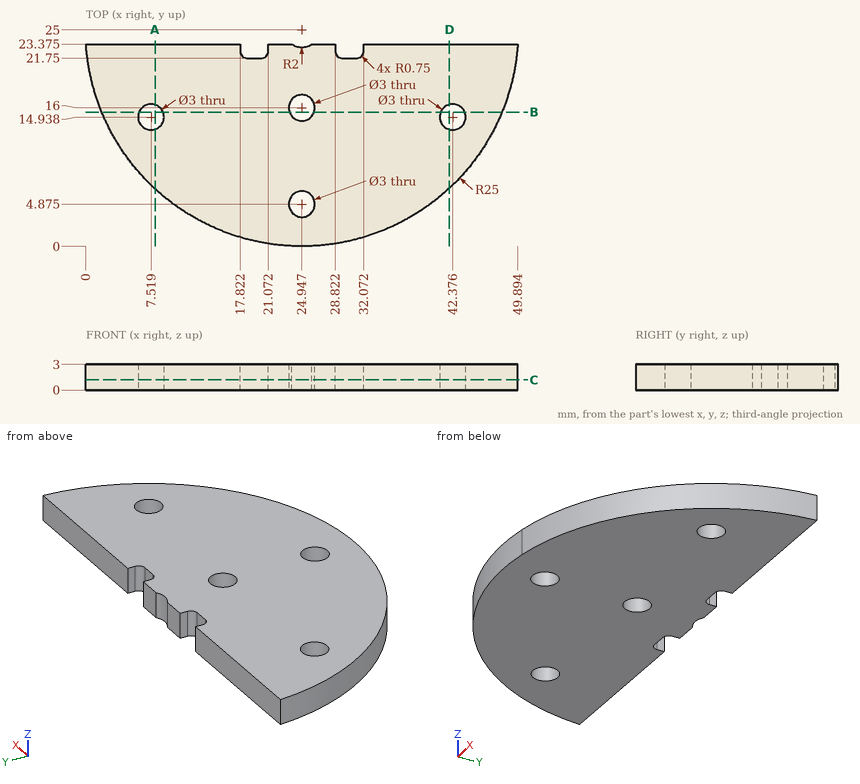
Here's the drawing with two shaded views (mm, measured from the low corner). I have some questions. Give positions to 0.01 mm unless a question says otherwise; leave off trailing zeros. Loops run counter-clockwise (first coordinate to the right, second up) from the corner with the lowest first, then second, coordinate; pieces in that order, holes last. Notation, with made-up numbers: (45.25, 13) -> (86.25, 13) arc R23 cw to (86.25, 28) -> close; hole circle Ø6 at (29, 77). An arc over 180 degrees is marked (long way). Answer as a JSON object with one key per item and string values. Group by question number.
Item 1: Imagine slicing it at B-B on y = 15.5. Write out the boundary of the cut face in (x, z) (1 decimal).
Item 2: Imagine slicing it at D-D on x = 42. Write out the boundary of the cut face in (y, z) (1 decimal).
Item 3: Imagine slicing it at A-A on x = 8. Write out the boundary of the cut face in (y, z) (1 decimal).
Item 4: I need wall thicknesses on L1, parallel to Y at x = 25, z = 2.7 (1 decimal); L2, parallel to X at y = 22, z = 2.6 (1 decimal); L3, parallel to Y at x = 42.5, z = 1.7 (1 decimal). Which ranges of each line are inside material? Lowest first, please.
Item 5: Imagine slicing it at C-C on z = 1.2. Give the number of separate pieces and of enclosed holes in the cut face.
Item 6: Will these pins go through, and if not, where does the flat tip stop? pin 1 (1 mm diameter, centred on x = 25, z = 2.5, fed in from +Y); pin 2 (0.7 mm diameter, centred on y = 23, z = 1, fed in from -X); pin 3 (3.5 mm diameter, centred on x = 24.95, y = 16, fed in from +Z); pin 4 (0.9 mm diameter, centred on x = 20, z = 1, fed in from +Y).
Answer list:
{
 "1": {"outline": "(1.8, 0) -> (6.1, 0) -> (6.1, 3) -> (1.8, 3) -> close; (8.9, 0) -> (23.5, 0) -> (23.5, 3) -> (8.9, 3) -> close; (26.4, 0) -> (41, 0) -> (41, 3) -> (26.4, 3) -> close; (43.8, 0) -> (48.1, 0) -> (48.1, 3) -> (43.8, 3) -> close"},
 "2": {"outline": "(6.7, 0) -> (13.5, 0) -> (13.5, 3) -> (6.7, 3) -> close; (16.4, 0) -> (23.4, 0) -> (23.4, 3) -> (16.4, 3) -> close"},
 "3": {"outline": "(6.6, 0) -> (13.5, 0) -> (13.5, 3) -> (6.6, 3) -> close; (16.4, 0) -> (23.4, 0) -> (23.4, 3) -> (16.4, 3) -> close"},
 "4": {"L1": "y = 0 to 3.4, 6.4 to 14.5, 17.5 to 23", "L2": "x = 0.1 to 18, 20.9 to 29, 31.9 to 49.8", "L3": "y = 7.2 to 13.4, 16.4 to 23.4"},
 "5": {"separate pieces": "1", "enclosed holes": "4"},
 "6": {"pin 1": "stops at y = 23.08", "pin 2": "stops at x = 0", "pin 3": "stops at z = 3", "pin 4": "stops at y = 21.76"}
}
